```python
from build123d import *

# Parameters (mm, degrees)
BOSS_EXTRUDE1_DEPTH = 1.5875
SKETCH2_R           = 6.74878
SKETCH2_R_2         = 3.96875
SKETCH2_W           = 12.7
SKETCH2_H           = 12.7
CUT_EXTRUDE1_DEPTH  = 1.5875
SKETCH3_R           = 1.0922
CUT_EXTRUDE2_DEPTH  = 64.189671282


with BuildPart() as part:
    # Sketch1 → Boss-Extrude1 (new body)
    with BuildSketch(Plane.XY):
        with BuildLine():
            Line((-52.840313991, 24.357951008), (55.109686009, 24.357951008))
            ThreePointArc((55.109686009, 24.357951008), (57.354750039, 23.428015038), (58.284686009, 21.182951008))
            Line((58.284686009, 21.182951008), (58.284686009, -10.567048992))
            ThreePointArc((58.284686009, -10.567048992), (57.354750039, -12.812113022), (55.109686009, -13.742048992))
            Line((55.109686009, -13.742048992), (-52.840313991, -13.742048992))
            ThreePointArc((-52.840313991, -13.742048992), (-55.085378022, -12.812113022), (-56.015313991, -10.567048992))
            Line((-56.015313991, -10.567048992), (-56.015313991, 21.182951008))
            ThreePointArc((-56.015313991, 21.182951008), (-55.085378022, 23.428015038), (-52.840313991, 24.357951008))
        make_face()
    extrude(amount=BOSS_EXTRUDE1_DEPTH)

    # Sketch2 → Cut-Extrude1 (cut)
    with BuildSketch(Plane(origin=(0, 0, 0), x_dir=(-1, 0, 0), z_dir=(0, 0, -1))):
        with Locations((16.645313991, 2.607931008)):
            Circle(SKETCH2_R)
        with Locations((-3.992186009, 2.607931008)):
            Circle(SKETCH2_R)
        with Locations((-24.629686009, 2.607931008)):
            Circle(SKETCH2_R)
        with Locations((-45.267186009, 2.607931008)):
            Circle(SKETCH2_R)
        with Locations((48.395313991, -1.042048992)):
            Circle(SKETCH2_R_2)
        with Locations((34.425313991, -1.042048992)):
            Rectangle(SKETCH2_W, SKETCH2_H)
    extrude(amount=-CUT_EXTRUDE1_DEPTH, mode=Mode.SUBTRACT)

    # Sketch3 → Cut-Extrude2 (cut, through all)
    with BuildSketch(Plane.XY.offset(1.5875)):
        with Locations((-16.645313991, 12.00793098)):
            Circle(SKETCH3_R)
        with Locations((3.989686009, 12.00793098)):
            Circle(SKETCH3_R)
        with Locations((24.624686009, 12.00793098)):
            Circle(SKETCH3_R)
        with Locations((-25.145314009, -1.44206902)):
            Circle(SKETCH3_R)
        with Locations((-4.510314009, -1.44206902)):
            Circle(SKETCH3_R)
        with Locations((33.124685991, -1.44206902)):
            Circle(SKETCH3_R)
        with Locations((45.259686009, 12.00793098)):
            Circle(SKETCH3_R)
        with Locations((53.759685991, -1.44206902)):
            Circle(SKETCH3_R)
    extrude(amount=-CUT_EXTRUDE2_DEPTH, mode=Mode.SUBTRACT)


solid = part.part
```
The listing builds one solid part. Answer for the finished solid, in the listing's coordinates (mm). Coordinates: 2 decimals unless noted, no trailing zeros. Write each loop counter-clockwise with the first axis right and the second up, starting at its lowest first coordinate (ties: lowest second). Pieces come first, ordered by that corner, then holes. Notation, with made-up numbers: M -27,29 L -3,29 A21 ccw -3,58 Z; hole C 0.5,52 d8. An arc over 180 degrees is marked long. Use a Markdown table: item, result. Add a question column.
1. Straight lines are drawn through the part: line 1 along Y through (x, z) = (-16.5, 0.7); line 2 along X through (y, z) = (6, 1.3); line 3 along Y through (x, z) = (-48, 0.85). For each, find the intervals that lie inside material, in ascending order. Write a range as [from, to].
2. Section B-B (x = -4.5) is taken. Give the vertices of the cut face in (y, z).
3. Section D-D (y = 7) is taken. Give the vertices of the cut face in (x, z).
4. Section C-C (z = 0.35) is taken. Count the separate pieces of the cut face and the enclosed holes in it, plus the area to 3 significant figures.
5. For a pull along Y with two mould halves and no side action, classify faces 1 (the cylindrical face through (-23.08, 4.64, 0.78)), 2 (the cylindrical face through (-55.11, 23.403, 0.783)), 3 (the flat face through (2, 10, 1.588)), 4 (the cylindrical face through (32.034, -1.394, 0.805)) as +Y half, -Y half, draft (parallel to the pull), parting line (faces both ways), or undercut.
6. Section A-A (y = -6) is taken. Give the vertices of the cut face in (x, z).
Data:
| question | item | result |
|---|---|---|
| 1 | line 1 | y = [-13.74, -4.14], [9.36, 10.93], [13.09, 24.36] |
| 1 | line 2 | x = [-56.02, -22.48], [-10.81, -1.84], [9.83, 18.8], [30.46, 39.43], [51.1, 58.28] |
| 1 | line 3 | y = [-13.74, -4.99], [2.91, 24.36] |
| 2 | outline | M -13.74,0 L -2.53,0 L -2.53,1.59 L -13.74,1.59 Z; M -0.35,0 L 24.36,0 L 24.36,1.59 L -0.35,1.59 Z |
| 3 | outline | M -56.02,0 L -21.77,0 L -21.77,1.59 L -56.02,1.59 Z; M -11.52,0 L -1.13,0 L -1.13,1.59 L -11.52,1.59 Z; M 9.12,0 L 19.51,0 L 19.51,1.59 L 9.12,1.59 Z; M 29.75,0 L 40.14,0 L 40.14,1.59 L 29.75,1.59 Z; M 50.39,0 L 58.28,0 L 58.28,1.59 L 50.39,1.59 Z |
| 4 | separate pieces | 1 |
| 4 | enclosed holes | 14 |
| 4 | area | 3,530 mm2 |
| 5 | face 1 | undercut |
| 5 | face 2 | +Y half |
| 5 | face 3 | draft |
| 5 | face 4 | undercut |
| 6 | outline | M -56.02,0 L -40.78,0 L -40.78,1.59 L -56.02,1.59 Z; M -28.08,0 L 58.28,0 L 58.28,1.59 L -28.08,1.59 Z |
